Design review of the part built by this model. Coordinates are the model's own, in mm. Face numbers are marked on the shaded views. A direction names the side the tool comes from. Coordinates: 2 decimals unless noted, no trailing zeros. Loops run counter-clockwise (first coordinate to the right, second up) from the corner with the lowest first, then second, coordinate; pieces in that order, holes last. Notation, with made-up numbers: (25, 30) - (64, 30) arc R17 ccw to (64, 56) - close; hole circle Ø5 at (69, -11). An arc over 180 degrees is marked (long way). One line per question, with ' | ' between items.
from build123d import *

# Parameters (mm, degrees)
SKETCH_1_R           = 40
EXTRUDE_1_DEPTH      = 110
SKETCH_2_R           = 3
CUT_EXTRUDE_2_DEPTH  = 150
SKETCH_3_R           = 50
CUT_EXTRUDE_3_DEPTH  = 50
CUT_EXTRUDE_4_DEPTH  = 10
SKETCH_5_W           = 36
SKETCH_5_H           = 160
CUT_EXTRUDE_7_DEPTH  = 122
CUT_EXTRUDE_8_DEPTH  = 10
SKETCH_7_R           = 3
CUT_EXTRUDE_9_DEPTH  = 10
EXTRUDE_START        = 4.3
EXTRUDE_2_DEPTH      = 4.3
SKETCH_11_W          = 36
SKETCH_11_H          = 48.823085464
SKETCH_11_R          = 3
EXTRUDE_3_DEPTH      = 4.3
CUT_EXTRUDE_START    = -200
CUT_EXTRUDE_16_DEPTH = 200
FILLET_2_R           = 1
CUT_EXTRUDE_START_2  = -25
CUT_EXTRUDE_17_DEPTH = 25
CUT_EXTRUDE_18_DEPTH = 100
SKETCH_17_R          = 100
CUT_EXTRUDE_19_DEPTH = 25
CUT_EXTRUDE_START_3  = -100
CUT_EXTRUDE_20_DEPTH = 100
SKETCH_19_W          = 186.41721719
SKETCH_19_H          = 278.516199491
CUT_EXTRUDE_21_DEPTH = 25
CUT_EXTRUDE_START_4  = 500
SKETCH_20_R          = 3
CUT_EXTRUDE_22_DEPTH = 500


with BuildPart() as part:
    # Sketch 1 → Extrude 1 (new body)
    with BuildSketch(Plane.XY):
        with BuildLine():
            Line((-100.092421442, 100), (199.907578558, 100))
            ThreePointArc((199.907578558, 100), (299.907578558, 0), (199.907578558, -100))
            Line((199.907578558, -100), (-100.092421442, -100))
            ThreePointArc((-100.092421442, -100), (-200.092421442, 0), (-100.092421442, 100))
        make_face()
        with Locations((-110.092421442, 0)):
            Circle(SKETCH_1_R, mode=Mode.SUBTRACT)
    extrude(amount=EXTRUDE_1_DEPTH)

    # Sketch 2 → Cut-Extrude 2 (cut)
    with BuildSketch(Plane(origin=(-100, 0, 0), x_dir=(0, 0, -1), z_dir=(1, 0, 0))):
        with Locations((-95, 0)):
            Circle(SKETCH_2_R)
        with Locations((-75, 0)):
            Circle(SKETCH_2_R)
        with Locations((-55, 0)):
            Circle(SKETCH_2_R)
    extrude(amount=-CUT_EXTRUDE_2_DEPTH, mode=Mode.SUBTRACT)

    # Sketch 3 → Cut-Extrude 3 (cut)
    with BuildSketch(Plane.XY.offset(110)):
        Circle(SKETCH_3_R)
    extrude(amount=-CUT_EXTRUDE_3_DEPTH, mode=Mode.SUBTRACT)

    # Sketch 4 → Cut-Extrude 4 (cut)
    with BuildSketch(Plane.XY.offset(60)):
        Polygon((36, 0), (18, 31.176914536), (-18, 31.176914536), (-36, 0), (-18, -31.176914536), (18, -31.176914536), align=None)
    extrude(amount=-CUT_EXTRUDE_4_DEPTH, mode=Mode.SUBTRACT)

    # Sketch 5 → Cut-Extrude 7 (cut)
    with BuildSketch(Plane.XY.offset(50)):
        Rectangle(SKETCH_5_W, SKETCH_5_H)
    extrude(amount=CUT_EXTRUDE_7_DEPTH, mode=Mode.SUBTRACT)

    # Sketch 6 → Cut-Extrude 8 (cut)
    with BuildSketch(Plane.XY.offset(50)):
        Polygon((36, 0), (18, 31.176914536), (-18, 31.176914536), (-36, 0), (-18, -31.176914536), (18, -31.176914536), align=None)
    extrude(amount=-CUT_EXTRUDE_8_DEPTH, mode=Mode.SUBTRACT)

    # Sketch 7 → Cut-Extrude 9 (cut)
    with BuildSketch(Plane.XY.offset(50)):
        with Locations((0, 62)):
            Circle(SKETCH_7_R)
    cut_extrude_9 = extrude(amount=-CUT_EXTRUDE_9_DEPTH, mode=Mode.SUBTRACT)

    # Mirror 1: Cut-Extrude 9 across plane
    add(cut_extrude_9.mirror(Plane.ZX), mode=Mode.SUBTRACT)

    # Sketch 10 → Extrude 2 (add)
    with BuildSketch(Plane.XY.offset(40).offset(EXTRUDE_START)):
        with BuildLine():
            ThreePointArc((18, 31.176914536), (31.176914536, 18), (36, 0))
            ThreePointArc((36, 0), (31.176914536, -18), (18, -31.176914536))
            Line((18, -31.176914536), (18, -46.647615159))
            ThreePointArc((18, -46.647615159), (41.231056256, -28.284271247), (50, 0))
            ThreePointArc((50, 0), (41.231056256, 28.284271247), (18, 46.647615159))
            Line((18, 46.647615159), (18, 31.176914536))
        make_face()
        with BuildLine():
            ThreePointArc((-36, 0), (-31.176914536, 18), (-18, 31.176914536))
            Line((-18, 31.176914536), (-18, 46.647615159))
            ThreePointArc((-18, 46.647615159), (-50, 0), (-18, -46.647615159))
            Line((-18, -46.647615159), (-18, -31.176914536))
            ThreePointArc((-18, -31.176914536), (-31.176914536, -18), (-36, 0))
        make_face()
        with BuildLine():
            Line((18, 31.176914536), (36, 0))
            ThreePointArc((36, 0), (31.176914536, 18), (18, 31.176914536))
        make_face()
        with BuildLine():
            ThreePointArc((18, -31.176914536), (31.176914536, -18), (36, 0))
            Line((36, 0), (18, -31.176914536))
        make_face()
        with BuildLine():
            ThreePointArc((-36, 0), (-31.176914536, -18), (-18, -31.176914536))
            Line((-18, -31.176914536), (-36, 0))
        make_face()
        with BuildLine():
            Line((-36, 0), (-18, 31.176914536))
            ThreePointArc((-18, 31.176914536), (-31.176914536, 18), (-36, 0))
        make_face()
    extrude(amount=-EXTRUDE_2_DEPTH)

    # Sketch 11 → Extrude 3 (add)
    with BuildSketch(Plane.XY.offset(50).offset(EXTRUDE_START)):
        with Locations((0, 55.588457268)):
            Rectangle(SKETCH_11_W, SKETCH_11_H)
        with Locations((0, 62)):
            Circle(SKETCH_11_R, mode=Mode.SUBTRACT)
    extrude_3 = extrude(amount=-EXTRUDE_3_DEPTH)

    # Mirror 4: Extrude 3 across plane
    add(extrude_3.mirror(Plane.ZX))

    # Sketch 14 → Cut-Extrude 16 (cut)
    with BuildSketch(Plane.XY.offset(110).offset(CUT_EXTRUDE_START)):
        with BuildLine():
            ThreePointArc((-114.938685096, -98.891801761), (-178.67776032, 0), (-114.938685096, 98.891801761))
            ThreePointArc((-114.938685096, 98.891801761), (-200.092421442, 0), (-114.938685096, -98.891801761))
        make_face()
    extrude(amount=CUT_EXTRUDE_16_DEPTH, mode=Mode.SUBTRACT)

    # Fillet 2
    fillet_2_edges = [part.edges().sort_by_distance(p)[0] for p in [
        (-50, 0, 110),
        (50, 0, 110),
        (0, -80, 110),
        (-18, 46.647615159, 85),
        (-18, -46.647615159, 85),
        (-18, -63.323807579, 110),
        (18, -46.647615159, 85),
        (18, 46.647615159, 85),
        (18, -63.323807579, 110),
        (-18, 63.323807579, 110),
        (18, 63.323807579, 110),
    ]]
    fillet(fillet_2_edges, radius=FILLET_2_R)

    # Sketch 15 → Cut-Extrude 17 (cut)
    with BuildSketch(Plane.XY.offset(110).offset(CUT_EXTRUDE_START_2)):
        with BuildLine():
            Line((199.907578558, 100), (199.907578558, -100))
            ThreePointArc((199.907578558, -100), (299.907578558, 0), (199.907578558, 100))
        make_face()
    cut_extrude_17 = extrude(amount=CUT_EXTRUDE_17_DEPTH, mode=Mode.SUBTRACT)

    # Mirror 5: Cut-Extrude 17 across plane
    add(cut_extrude_17.mirror(Plane.XY.offset(55)), mode=Mode.SUBTRACT)

    # Sketch 16 → Cut-Extrude 18 (cut)
    with BuildSketch(Plane.XY.offset(85)):
        with BuildLine():
            ThreePointArc((279.907578558, 0), (249.907578558, 30), (219.907578558, 0))
            Line((219.907578558, 0), (279.907578558, 0))
        make_face()
        with BuildLine():
            Line((279.907578558, 0), (219.907578558, 0))
            ThreePointArc((219.907578558, 0), (249.907578558, -30), (279.907578558, 0))
        make_face()
        with BuildLine():
            ThreePointArc((279.907578558, 0), (249.907578558, 30), (219.907578558, 0))
            Line((219.907578558, 0), (279.907578558, 0))
        make_face()
        with BuildLine():
            Line((279.907578558, 0), (219.907578558, 0))
            ThreePointArc((219.907578558, 0), (249.907578558, -30), (279.907578558, 0))
        make_face()
    extrude(amount=-CUT_EXTRUDE_18_DEPTH, mode=Mode.SUBTRACT)

    # Sketch 17 → Cut-Extrude 19 (cut)
    with BuildSketch(Plane.XY.offset(110).offset(CUT_EXTRUDE_START_2)):
        with Locations((199.907578558, 0)):
            Circle(SKETCH_17_R)
    cut_extrude_19 = extrude(amount=CUT_EXTRUDE_19_DEPTH, mode=Mode.SUBTRACT)

    # Mirror 6: Cut-Extrude 19 across plane
    add(cut_extrude_19.mirror(Plane.XY.offset(55)), mode=Mode.SUBTRACT)

    # Sketch 18 → Cut-Extrude 20 (cut)
    with BuildSketch(Plane.XY.offset(85).offset(CUT_EXTRUDE_START_3)):
        with BuildLine():
            ThreePointArc((272.856353648, 68.399387519), (284.723437561, 35.110699351), (288.748761353, 0))
            ThreePointArc((288.748761353, 0), (284.723437561, -35.110699351), (272.856353648, -68.399387519))
            ThreePointArc((272.856353648, -68.399387519), (299.907578558, 0), (272.856353648, 68.399387519))
        make_face()
    extrude(amount=CUT_EXTRUDE_20_DEPTH, mode=Mode.SUBTRACT)

    # Sketch 19 → Cut-Extrude 21 (cut)
    with BuildSketch(Plane.XY.offset(110)):
        with Locations((187.913249079, -8.044790623)):
            Rectangle(SKETCH_19_W, SKETCH_19_H)
    cut_extrude_21 = extrude(amount=-CUT_EXTRUDE_21_DEPTH, mode=Mode.SUBTRACT)

    # Mirror 7: Cut-Extrude 21 across plane
    add(cut_extrude_21.mirror(Plane.XY.offset(55)), mode=Mode.SUBTRACT)

    # Sketch 20 → Cut-Extrude 22 (cut)
    with BuildSketch(Plane(origin=(230, 0, 0), x_dir=(0, 0, -1), z_dir=(1, 0, 0)).offset(CUT_EXTRUDE_START_4)):
        with Locations((-55, 0)):
            Circle(SKETCH_20_R)
        with Locations(Location((-55, 15, 0), (0, 0, 180))):
            Circle(SKETCH_20_R)
        with Locations(Location((-55, -15, 0), (0, 0, 180))):
            Circle(SKETCH_20_R)
    extrude(amount=-CUT_EXTRUDE_22_DEPTH, mode=Mode.SUBTRACT)


solid = part.part
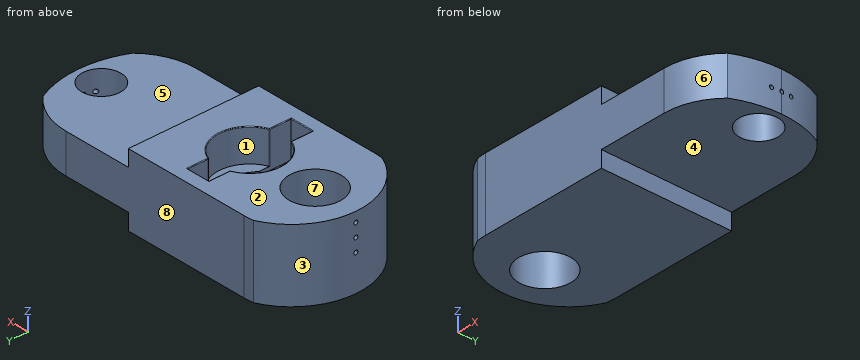
Q1. For pin 1 (6 mm diameter, centred on x = 168, y = -32.5, fed in from -Z); pin 2 (2 mm diameter, centred on x = 8, y = -52, fed in from +Z); pin 3 (3 mm diameter, centred on y = 18.5, z = 46, fed in from -X); pin 4 (8 mm diameter, centred on y = 0, z = 95, fed in from -X), all flat-tipped, find the tip position at first contact; note any pin that passes through.
Returned:
pin 1: stops at z = 25 | pin 2: stops at z = 54.3 | pin 3: stops at x = -177.34 | pin 4: stops at x = -178.68
Q2. Take a section at B-B (y = -54). Give the boundary of the cut face in (x, z), plus the area to 3 significant figures.
Returned:
outline: (-164.3, 0) - (94.7, 0) - (94.7, 25) - (279.05, 25) - (279.05, 85) - (94.7, 85) - (94.7, 110) - (19, 110) arc R1 ccw to (18, 109) - (18, 54.3) - (-18, 54.3) - (-18, 109) arc R1 ccw to (-19, 110) - (-164.3, 110) - close | area: 37,500 mm²
Q3. Take a section at A-A (z = 14). Give the boundary of the cut face in (x, y).
Returned:
outline: (-114.94, -98.89) arc R100 ccw to (-100.09, -100) - (94.7, -100) - (94.7, 100) - (-100.09, 100) arc R100 ccw to (-114.94, 98.89) arc R108.59 ccw to start; hole circle Ø80 at (-110.09, 0)
Q4. Draft analysis for pull direction Y (two halves, no side actions). For the marked faces 6, 7 and 8, state which applies: +Y half, -Y half, draft (parallel to the pull), parting line (faces both ways), or undercut.
Returned:
face 6: -Y half | face 7: undercut | face 8: +Y half
Q5. Tool access review of the marked faces 1, 2, 3, 4 and 5: name each direction out of +Z, -Z, +X, -X, +Y, -Y from which nothing blocks a thin tool from reaching the whole face with its end or side.
Returned:
face 1: +Z | face 2: +Z, +X, -X, +Y, -Y | face 3: +Z, -Z, -X | face 4: -Z, +X, +Y, -Y | face 5: +Z, +X, +Y, -Y
Q6. Take a section at C-C (x = 150). Give the boundary of the cut face in (y, z).
Returned:
outline: (-100, 25) - (100, 25) - (100, 85) - (-100, 85) - close
Q7. To check wall thickness, follow line 1 along Z through (x, y) = (-157.75, 0); line 2 along Y through (x, z) = (0, 102); line 3 along X through (y, z) = (-19, 102.5). State the ranges of each line that lie inside material, in increasing order.
Returned:
line 1: z = 0 to 52, 58 to 72, 78 to 92, 98 to 110 | line 2: y = -100 to -80, 80 to 100 | line 3: x = -177 to -145.29, -74.89 to -46.25, 46.25 to 94.7
